CAD build for the part. Positions are in the model's coordinates, mm. Face numbers are marked on the shaded views. A direction names the side the tool comes from. Coordinates: 2 decimals unless noted, no trailing zeros. Write each loop counter-clockwise with the first axis right and the second up, starting at its lowest first coordinate (ties: lowest second). Pieces come first, ordered by that corner, then holes.
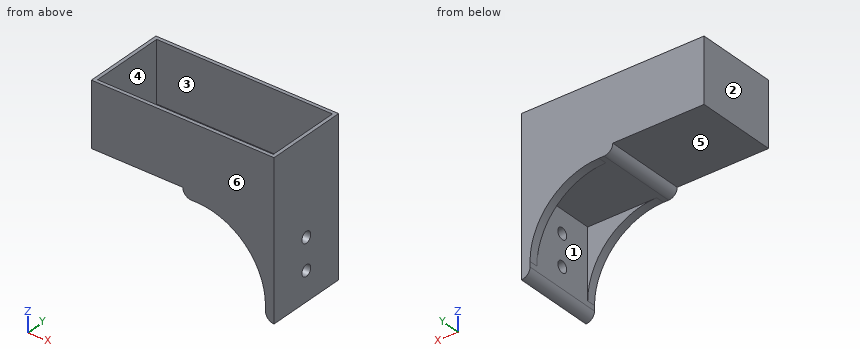
```python
from build123d import *

# Parameters (mm, degrees)
F0_W     = 106
F0_H     = 47.5
F0_W_2   = 102
F0_H_2   = 43.5
F1_DEPTH = 2
F2_W     = 106
F2_H     = 47.5
F2_W_2   = 102
F2_H_2   = 43.5
F3_DEPTH = 35
F5_DEPTH = 47.5
F6_W     = 37.5
F6_H     = 48
F7_DEPTH = 101
F8_R     = 3.25
F9_DEPTH = 25


with BuildPart() as f1:
    # F0 (on Top) → F1 (new body)
    with BuildSketch(Plane.XY):
        Rectangle(F0_W, F0_H)
        Rectangle(F0_W_2, F0_H_2, mode=Mode.SUBTRACT)
        Rectangle(F0_W_2, F0_H_2)
    extrude(amount=F1_DEPTH)

    # F2 (on face) → F3 (join)
    with BuildSketch(Plane.XY.offset(2)):
        Rectangle(F2_W, F2_H)
        Rectangle(F2_W_2, F2_H_2, mode=Mode.SUBTRACT)
    extrude(amount=F3_DEPTH)

    # F4 (on face) → F5 (join)
    with BuildSketch(Plane.XZ.offset(23.75)):
        with BuildLine():
            Line((53, -5), (53, 0))
            Line((53, 0), (0, 0))
            ThreePointArc((0, 0), (1.464466, -3.535534), (5, -5))
            Line((5, -5), (8, -5))
            ThreePointArc((8, -5), (36.284271, -16.715729), (48, -45))
            Line((48, -45), (48, -48))
            ThreePointArc((48, -48), (49.464466, -51.535534), (53, -53))
            Line((53, -53), (53, -5))
        make_face()
    extrude(amount=-F5_DEPTH)

    # F6 (on face) → F7 (cut)
    with BuildSketch(Plane(origin=(-53, 0, 0), x_dir=(0, -1, 0), z_dir=(-1, 0, 0))):
        with Locations((0, -29)):
            Rectangle(F6_W, F6_H)
    extrude(amount=-F7_DEPTH, mode=Mode.SUBTRACT)

    # F8 (on face) → F9 (cut)
    with BuildSketch(Plane(origin=(48, 0, 0), x_dir=(0, -1, 0), z_dir=(-1, 0, 0))):
        with Locations((0, -18)):
            Circle(F8_R)
        with Locations((0, -36)):
            Circle(F8_R)
    extrude(amount=-F9_DEPTH, mode=Mode.SUBTRACT)


solid = f1.part
```
Item 1: Which spindle directions (+Z, -Z, +X, -X, +Y, -Y) get a long thin tool onto all of the face, cutting with end or side? Do the marked faces 1, 2 and 3. Say none if no direction does.
Item 2: Saw through at B-B, the plane x = -6. Write the cut outline in (y, z), and give its area (3 significant figures).
Item 3: Saw through at A-A, the plane z = 21. Write the cut outline in (x, y).
Item 4: Saw through at C-C, the plane y = 0. Write the cut outline in (x, z), and give its area (3 significant figures).
Item 5: Flat gauge pins, fed straight in: pin 1 Ø13 at (x, y) = (24, 2.5) entering from +Z; pin 2 Ø14 at (x, y) = (-17.5, 11.5) entering from -Z; pin 3 Ø8 at (y, z) = (-14, -36.5) entering from -X; pin 4 Ø6 at (y, z) = (0, -18) entering from -X. Where does each tip first touch, or does it go through?
Item 6: Wall check: line 1 along Z through (x, y) = (49, 0); line 2 along Z through (x, y) = (49.65, 0); line 3 along Y through (x, z) = (44, -19). Give the ranges that are in metal, low to high.
Item 7: Saw through at D-D, the plane z = -37.5. Write the cut outline in (x, y).
Item 8: Two-plate mould, pull along Y, no slides. Class the marked faces 4, 5 and 6: +Y half, -Y half, draft (parallel to the pull), parting line (faces both ways), or undercut.
Working result:
1. face 1: -Z, -X
1. face 2: +Z, -Z, -X, +Y, -Y
1. face 3: +Z
2. outline: (-23.75, 0) - (23.75, 0) - (23.75, 37) - (21.75, 37) - (21.75, 2) - (-21.75, 2) - (-21.75, 37) - (-23.75, 37) - close
2. area: 235 mm2
3. outline: (-53, -23.75) - (53, -23.75) - (53, 23.75) - (-53, 23.75) - close; hole (-51, -21.75) - (51, -21.75) - (51, 21.75) - (-51, 21.75) - close
4. outline: (-53, 0) - (0, 0) arc R5 ccw to (5, -5) - (48, -5) - (48, -14.75) - (53, -14.75) - (53, 37) - (51, 37) - (51, 2) - (-51, 2) - (-51, 37) - (-53, 37) - close; (48, -48) arc R5 ccw to (53, -53) - (53, -39.25) - (48, -39.25) - close; (48, -32.75) - (53, -32.75) - (53, -21.25) - (48, -21.25) - close
4. area: 781 mm2
5. pin 1: stops at z = 2
5. pin 2: stops at z = 0
5. pin 3: stops at x = 48
5. pin 4: passes through
6. line 1: z = -51 to -39.25, -32.75 to -21.25, -14.75 to 2
6. line 2: z = -51.71 to -39.25, -32.75 to -21.25, -14.75 to 2
6. line 3: y = -23.75 to -18.75, 18.75 to 23.75
7. outline: (47.29, -23.75) - (53, -23.75) - (53, -2.88) - (48, -2.88) - (48, -18.75) - (47.29, -18.75) - close; (47.29, 18.75) - (48, 18.75) - (48, 2.88) - (53, 2.88) - (53, 23.75) - (47.29, 23.75) - close
8. face 4: undercut
8. face 5: draft
8. face 6: -Y half
